Autodesk Inventor part; units mm, degrees
ref_plane "YZ Plane" through (0, 0, 0) normal (1, 0, 0) x (0, 1, 0)
ref_plane "XZ Plane" through (0, 0, 0) normal (0, 1, 0) x (-1, 0, 0)
ref_plane "XY Plane" through (0, 0, 0) normal (0, 0, 1) x (1, 0, 0)
sketch "Эскиз1" plane through (0, 0, 0) normal (0, 0, 1) x (1, 0, 0)
  line L0 (62, -18) -> (62, 0)
  line L1 (62, 0) -> (0, 0)
  line L2 (62, 0) -> (0, 0)
  line L3 (62, -18) -> (15, -18)
  line L4 (0, 0) -> (0, -38)
  line L5 (0, -38) -> (15, -38)
  line L6 (15, -38) -> (15, -18)
  dimension "d27" = 18
  dimension "d32" = 62
  dimension "d40" = 20
  dimension "d41" = 15
  dimension "d42" = 38
extrude "Выдавливание1" add sketch "Эскиз1" along normal blind 15
sketch "Эскиз2" plane through (0, 0, 0) normal (0, 0, -1) x (-1, 0, 0)
  circle A0 centre (-7.6337, -29.0677) radius 2.1
  point P0 (0, 0)
  dimension "d37" = 4.2
extrude "Выдавливание2" cut sketch "Эскиз2" against normal through all
sketch "Эскиз3" plane through (0, 0, 15) normal (0, 0, 1) x (1, 0, 0)
  line L0 (62, 0) -> (0, 0)
  line L1 (0, 0) -> (10, 0)
  line L2 (10, 0) -> (10, -20)
  line L3 (10, -20) -> (0, -20)
  line L4 (0, -20) -> (0, 0)
  point P0 (10, 0)
  dimension "d7" = 20
  dimension "d8" = 10
extrude "Выдавливание3" add sketch "Эскиз3" along normal blind 18.5
mirror "Зеркальное отражение1" about plane through (5, -10, 33.5) normal (0, 0, 1)
sketch "Эскиз6" plane through (0, 0, 0) normal (0, 1, 0) x (1, 0, 0)
  circle A0 centre (5.333, -60.2954) radius 1.5
  circle A1 centre (18.6772, -7.9811) radius 1.5
  circle A2 centre (18.6772, -60.2954) radius 1.5
  circle A3 centre (5.333, -7.9811) radius 1.5
  circle A4 centre (34.4058, -60.2954) radius 1.5
  circle A5 centre (34.4058, -7.9811) radius 1.5
  circle A6 centre (56.8865, -7.9811) radius 1.5
  circle A7 centre (56.8865, -60.2954) radius 1.5
  point P0 (0, 0)
  dimension "d21" = 3
  dimension "d22" = 3
  dimension "d23" = 3
  dimension "d24" = 3
  dimension "d33" = 3
  dimension "d34" = 3
  dimension "d35" = 3
  dimension "d36" = 3
extrude "Выдавливание6" cut sketch "Эскиз6" against normal blind 13
sketch "Эскиз7" plane through (0, 0, 0) normal (0, 1, 0) x (1, 0, 0)
  line L0 (62, 0) -> (62, -15)
  line L1 (62, -15) -> (62, -12.4939)
  line L2 (11.1046, -12.4939) -> (11.1046, -15)
  line L3 (62, -15) -> (10, -15)
  line L4 (62, -15) -> (11.1046, -15)
  line L5 (11.1046, -12.4939) -> (62, -12.4939)
  point P0 (0, 0)
extrude "Выдавливание7" cut sketch "Эскиз7" against normal blind 10
sketch "Эскиз8" plane through (0, -38, 0) normal (-1, 0, 0) x (0, 0, 1)
  point P0 (0, 38)
ref_plane "РабПлоскость3" through (0, 0, 35.5) normal (0, 0, 1) x (1, 0, 0)
ref_plane "РабПлоскость2" through (0, 0, 33.5) normal (0, 0, 1) x (1, 0, 0)
sketch "Эскиз9" plane through (0, 0, 35.5) normal (0, 0, 1) x (1, 0, 0)
  line L0 (0, 0) -> (0, -38)
  circle A0 centre (-10.4982, -19.8582) radius 5
  line L1 (0, -20) -> (0, -38)
  line L2 (0, -14.2319) -> (0, -12.6158)
  circle A1 centre (-10.4982, -19.8582) radius 2.1
  line L3 (0, -12.6158) -> (0, -14.2319)
  line L4 (-13.4667, -15.8348) -> (1.5377, -4.7644)
  line L5 (-6.9627, -23.3937) -> (0, -16.431)
  line L6 (0, -5.899) -> (0, -16.431)
  point P0 (-15.4732, -20.3581)
  point P1 (-12.5479, -24.4188)
  point P2 (0, -3.6635)
  dimension "d46" = 4.2
  dimension "d47" = 10
  dimension "d52" = 45
extrude "Выдавливание8" add sketch "Эскиз9" along normal blind 4
mirror "Зеркальное отражение2" about plane through (0, 0, 33.5) normal (0, 0, 1) of "Выдавливание8"
properties part number "кроншейн"
Geometry: final body of the model. Coordinates: model frame, mm. A direction names the side the tool comes from. Round coordinates to 2 decimals unless told otherwise and drop trailing zeros. Order: outer loops, then holes, each group sorted by start corner. A loop starts at its lowest first (then second) coordinate and runs counter-clockwise, first axis right, second up. Notation, with made-up numbers: (1, -4) -> (14, -4) arc R27 cw to (14, 34) -> close; hole circle Ø3 at (64.25, 82.25). An arc over 180 degrees is marked (long way). Put each result on its own line as item: value. Start each with the question number.
Q1. Section C-C on z = 56. Return the cut outline in (x, y), and give its area (3 significant figures).
Q2. Section B-B on x = 26.5. Return the cut outline in (y, z), and give its area (3 significant figures).
Q3. Line query: probe 1 along Z at (x, y) = (10.5, -2.5); probe 2 along Z at (x, y) = (55, -5); probe 3 along X at (y, z) = (-9, 59.5). Output: solid intervals per line, ascending.
Q4. Section D-D on y = -3.5. Give the number of separate pieces and of enclosed holes in the cut face, and give its area (3 significant figures).
Q5. Pull-direction query (Y, two-part tool) for faces 4 (the flat face through (-3.53, -19.96, 37.47)), 5 (the cylindrical face through (8.089, -31.118, 7.395)), 6 (the flat face through (36, -10, 14)), 7 (the flat face through (25, -10, 67)); classes: +Y half, -Y half, draft (parallel to the pull), parting line (faces both ways), or undercut.
Q6. First-contact query: pin 1 (2.5 mm diameter, centred on x = 56.89, z = 7.98, fed in from +Y); pin 2 (4.5 mm diameter, centred on x = 46.5, z = 56.5, fed in from -Y); pin 3 (16.5 mm diameter, centred on y = -33, z = 57.5, fed in from +X). Flat tips, straight axial feed; report the tip coordinate or a pass-through.
Q7. Section A-A on y = -34. Return the cut outline in (x, z), and give its area (3 significant figures).
Q8. Reachability of faces 1 (the flat face through (-8, -17, 27.5)), 2 (the flat face through (-6, -17, 39.5)), 3 (the cylindrical face through (33.3, -6.41, 6.97)) from +Z, -Z, +X, -X, +Y, -Y: full face, straight path, thin tool, end or side. Return the list, or none.
Ans:
1. outline: (0, -38) -> (15, -38) -> (15, -18) -> (62, -18) -> (62, 0) -> (0, 0) -> close; hole circle Ø4.2 at (7.63, -29.07)
1. area: 1,400 mm2
2. outline: (-18, 0) -> (0, 0) -> (0, 12.49) -> (-10, 12.49) -> (-10, 15) -> (-18, 15) -> close; (-18, 52) -> (0, 52) -> (0, 67) -> (-18, 67) -> close
2. area: 515 mm2
3. probe 1: z = 0 to 15, 52 to 67
3. probe 2: z = 0 to 12.49, 52 to 67
3. probe 3: x = 0 to 4.06, 6.6 to 17.41, 19.95 to 33.13, 35.68 to 55.61, 58.16 to 62
4. separate pieces: 1
4. enclosed holes: 8
4. area: 2,050 mm2
5. face 4: -Y half
5. face 5: undercut
5. face 6: +Y half
5. face 7: draft
6. pin 1: stops at y = -13
6. pin 2: stops at y = -18
6. pin 3: stops at x = 15
7. outline: (0, 0) -> (15, 0) -> (15, 15) -> (0, 15) -> close; (0, 52) -> (15, 52) -> (15, 67) -> (0, 67) -> close
7. area: 450 mm2
8. face 1: -Z, -X, +Y, -Y
8. face 2: +Z, -X, +Y, -Y
8. face 3: +Y
